The figure shows three views and two pictorial views of one solid part (mm, origin at its lowest corner). Answer the questions. A direction names the side the tool comes from. Coordinates: 2 decimals unless noted, no trailing zeros. Write each loop counter-clockwise with the first axis right and the second up, starting at its lowest first coordinate (ties: lowest second). Pieces come first, ordered by that corner, then holes.
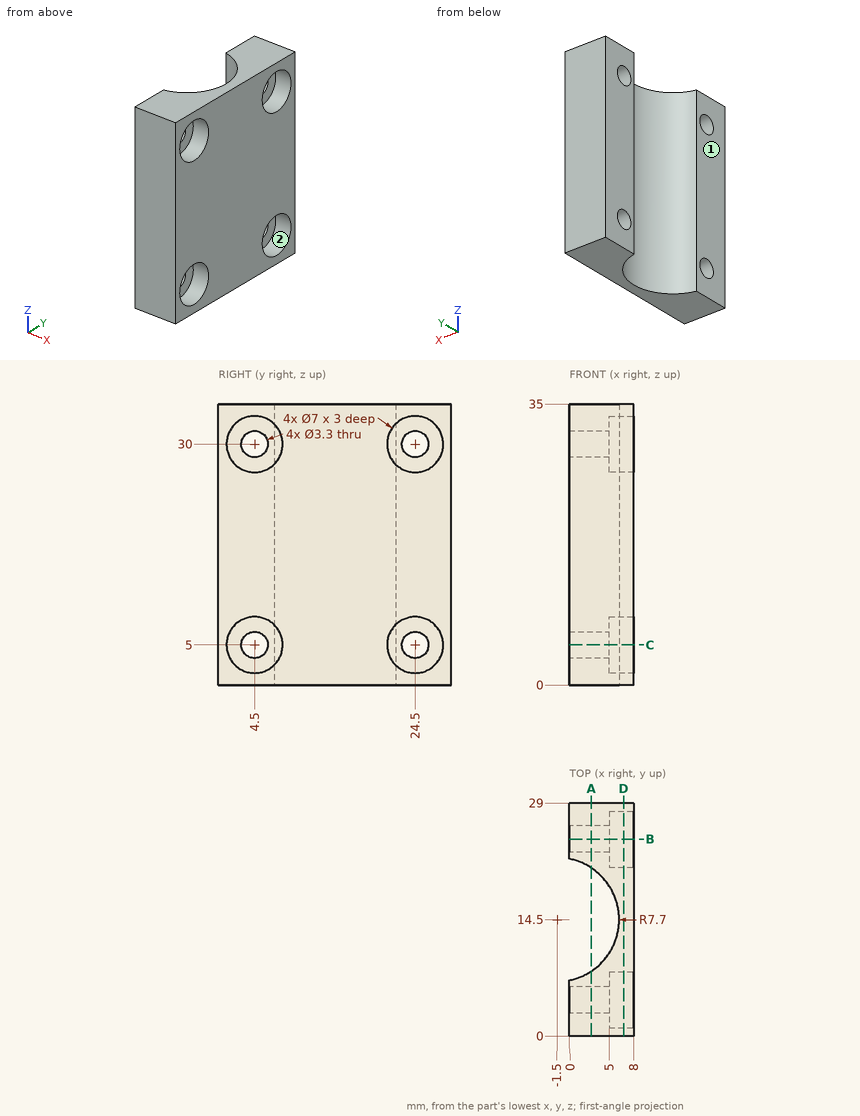
Q1. The part is cut by section D-D, the plane x = 6.75. Write down the section's boundary in (y, z), then the cut area to 3 significant figures.
Answers below:
outline: (0, 0) - (29, 0) - (29, 35) - (0, 35) - close; hole circle Ø7 at (4.5, 5); hole circle Ø7 at (4.5, 30); hole circle Ø7 at (24.5, 5); hole circle Ø7 at (24.5, 30)
area: 861 mm2
Q2. The part is cut by section C-C, the plane z = 5. Write down the section's boundary in (x, y), then the cut area to 3 significant figures.
Answers below:
outline: (0, 0) - (8, 0) - (8, 1) - (5, 1) - (5, 2.85) - (0, 2.85) - close; (0, 6.15) - (5, 6.15) - (5, 8) - (8, 8) - (8, 21) - (5, 21) - (5, 22.85) - (0, 22.85) - (0, 22.05) arc R7.7 cw to (0, 6.95) - close; (0, 26.15) - (5, 26.15) - (5, 28) - (8, 28) - (8, 29) - (0, 29) - close
area: 86.8 mm2
Q3. Given pin 1 (4 mm diameter, centred on y = 24.5, z = 5, fed in from +X), flat-ended and moving along its own axis, determine where the tip first touches the part or whether it passes through.
Answers below:
pin 1: stops at x = 5
Q4. Which of the six approach directions +Z, -Z, +X, -X, +Y, -Y give full straight-line access (tool end or side, diameter ignored) to the marked faces 1 and 2?
Answers below:
face 1: +Z, -Z, -X, +Y, -Y
face 2: +X
Q5. The part is cut by section B-B, the plane y = 24.5. Write down the section's boundary in (x, z).
Answers below:
outline: (0, 0) - (8, 0) - (8, 1.5) - (5, 1.5) - (5, 3.35) - (0, 3.35) - close; (0, 6.65) - (5, 6.65) - (5, 8.5) - (8, 8.5) - (8, 26.5) - (5, 26.5) - (5, 28.35) - (0, 28.35) - close; (0, 31.65) - (5, 31.65) - (5, 33.5) - (8, 33.5) - (8, 35) - (0, 35) - close
Q6. The part is cut by section A-A, the plane x = 2.75. Write down the section's boundary in (y, z), then the cut area to 3 significant figures.
Answers below:
outline: (0, 0) - (8.08, 0) - (8.08, 35) - (0, 35) - close; (20.92, 0) - (29, 0) - (29, 35) - (20.92, 35) - close; hole circle Ø3.3 at (4.5, 5); hole circle Ø3.3 at (4.5, 30); hole circle Ø3.3 at (24.5, 5); hole circle Ø3.3 at (24.5, 30)
area: 531 mm2
Q7. Find the intervals of material crossed by probe 1 along Y at (x, z) = (7.2, 30); probe 2 along Y at (x, z) = (3.15, 30); probe 3 along Z at (x, y) = (2.25, 24.25), in increasing order.
Answers below:
probe 1: y = 0 to 1, 8 to 21, 28 to 29
probe 2: y = 0 to 2.85, 6.15 to 8.36, 20.64 to 22.85, 26.15 to 29
probe 3: z = 0 to 3.37, 6.63 to 28.37, 31.63 to 35
